Work out the finished part from the listing and answer in its coordinate system (mm). A direction names the side the tool comes from. Round coordinates to 2 decimals unless told otherwise and drop trailing zeros. Write each loop counter-clockwise with the first axis right and the second up, starting at its lowest first coordinate (ties: lowest second). Pieces come first, ordered by that corner, then holes. Notation, with made-up numbers: (43, 20) - (78, 20) arc R14 ccw to (78, 36) - close; hole circle Ø7 at (61.25, 37). An arc over 180 degrees is marked (long way). Answer as a JSON object with one key per item and string values.
```python
from build123d import *

# Parameters (mm, degrees)
SKETCH1_R           = 5.1
BOSS_EXTRUDE1_DEPTH = 10
SKETCH2_W           = 7.5
SKETCH2_H           = 16
BOSS_EXTRUDE2_DEPTH = 85
SKETCH3_W           = 29.2
SKETCH3_H           = 16
SKETCH3_R           = 5.1
BOSS_EXTRUDE3_DEPTH = 10
SKETCH4_W           = 29.2
SKETCH4_H           = 12
BOSS_EXTRUDE4_DEPTH = 10
CUT_EXTRUDE1_REACH  = 31.2
SKETCH6_W           = 29.2
SKETCH6_H           = 9.155809416
BOSS_EXTRUDE5_DEPTH = 28.3
SKETCH7_R           = 2.5
CUT_EXTRUDE2_DEPTH  = 20


with BuildPart() as part:
    # Sketch1 → Boss-Extrude1 (new body)
    with BuildSketch(Plane.XY):
        Polygon((-7.1, 8), (-14.6, 8), (-14.6, -8), (-7.1, -8), (7.1, -8), (14.6, -8), (14.6, 8), (7.1, 8), align=None)
        Circle(SKETCH1_R, mode=Mode.SUBTRACT)
    extrude(amount=BOSS_EXTRUDE1_DEPTH)

    # Sketch2 → Boss-Extrude2 (add)
    with BuildSketch(Plane.XY.offset(10)):
        with Locations((-10.85, 0)):
            Rectangle(SKETCH2_W, SKETCH2_H)
        with Locations((10.85, 0)):
            Rectangle(SKETCH2_W, SKETCH2_H)
    extrude(amount=BOSS_EXTRUDE2_DEPTH)

    # Sketch3 → Boss-Extrude3 (add)
    with BuildSketch(Plane.XY.offset(95)):
        Rectangle(SKETCH3_W, SKETCH3_H)
        Circle(SKETCH3_R, mode=Mode.SUBTRACT)
    extrude(amount=-BOSS_EXTRUDE3_DEPTH)

    # Sketch4 → Boss-Extrude4 (add)
    with BuildSketch(Plane.XY.offset(95)):
        with Locations((0, -14)):
            Rectangle(SKETCH4_W, SKETCH4_H)
    extrude(amount=-BOSS_EXTRUDE4_DEPTH)

    # Sketch5 → Cut-Extrude1 (cut, up to next)
    with BuildSketch(Plane(origin=(14.6, 0, 0), x_dir=(0, 0, -1), z_dir=(1, 0, 0)), mode=Mode.PRIVATE) as cut_extrude1_sk1:
        Polygon((-95, -12.5), (-89.748443463, -20), (-95, -20), align=None)
    cut_extrude1_tool1 = extrude(cut_extrude1_sk1.sketch, amount=-CUT_EXTRUDE1_REACH, mode=Mode.PRIVATE) & part.part
    add(cut_extrude1_tool1.solids().sort_by_distance((14.6, -17.5, 93.249481))[0], mode=Mode.SUBTRACT)

    # Sketch6 → Boss-Extrude5 (add)
    with BuildSketch(Plane(origin=(0, -48.747773592, 69.619035688), x_dir=(1, 0, 0), z_dir=(0, -0.573576436, 0.819152044))):
        with Locations((0, 39.672456192)):
            Rectangle(SKETCH6_W, SKETCH6_H)
    extrude(amount=BOSS_EXTRUDE5_DEPTH)

    # Sketch7 → Cut-Extrude2 (cut)
    with BuildSketch(Plane(origin=(0, -64.97998674, 92.801038541), x_dir=(1, 0, 0), z_dir=(0, -0.573576436, 0.819152044))):
        with Locations((-7.3, 39.672456192)):
            Circle(SKETCH7_R)
        with Locations((7.3, 39.672456192)):
            Circle(SKETCH7_R)
    extrude(amount=-CUT_EXTRUDE2_DEPTH, mode=Mode.SUBTRACT)


solid = part.part
```
Item 1: A cutting plane is placed at A-A (z = 68.5). Write down the section's boundary in (x, y), and give its area (3 significant figures).
Results found:
{"outline": "(-14.6, -8) - (-7.1, -8) - (-7.1, 8) - (-14.6, 8) - close; (7.1, -8) - (14.6, -8) - (14.6, 8) - (7.1, 8) - close", "area": "240 mm²"}
Item 2: Each of these flat-tipped pins is pushed along its axis until it touches: P1, Ø4, axis at x = -10, y = -21, coming from the +Z side; P2, Ø14.5, axis at x = -0.5, z = 39.5, coming from the -Y side; P3, Ø1.4, axis at x = -4, z = 88, coming from the -Y side; P4, Ø3, axis at x = -10, y = -6.5, coming from the -Z side. Where does it stop, or does it pass through?
Results found:
{"P1": "z = 110", "P2": "y = -8", "P3": "y = -20", "P4": "z = 0"}
Item 3: For faces 4 (the flat face through (7.1, 0, 47)), 5 (the flat face through (-10, 8, 47)), 6 (the flat face through (0, -9, 85)), 7 (the flat face through (-10, -8, 42)), 8 (the flat face through (-7.335, -20.982, 99.193)), determine the directions among +Z, -Z, +X, -X, +Y, -Y from which every point of the face is accessible in a straight line to the end or side of a thin tool.
Results found:
{"face 4": "+Y, -Y", "face 5": "+Z, -Z, +X, -X, +Y", "face 6": "-Y", "face 7": "-Z, +X, -X, -Y", "face 8": "none"}
Item 4: Determine the mould class of faces 1 (the flat face through (-0.204, -20.502, 106.429)), 2 (the cylindrical face through (2.4, -4.5, 90.1)), 3 (the flat face through (14.6, -2, 59)) for opening direction Y: pulls with the +Y half, pulls with the -Y half, needs draft (parallel to the pull), parting line crosses it, or undercut.
Results found:
{"face 1": "pulls with the +Y half", "face 2": "undercut", "face 3": "needs draft"}
Item 5: Consider line 1 along Z through (x, y) = (5.25, -3); line 2 along X through (y, z) = (3.5, 46); line 3 along Y through (x, z) = (0, 5.25). Determine where each line is inside the solid, lowest interval first.
Results found:
{"line 1": "0 to 10, 85 to 95", "line 2": "-14.6 to -7.1, 7.1 to 14.6", "line 3": "-8 to -5.1, 5.1 to 8"}
Item 6: A cutting plane is placed at D-D (z = 109). Give the number of separate pieces and of enclosed holes in the cut face, and give its area (3 significant figures).
Results found:
{"separate pieces": "1", "enclosed holes": "2", "area": "278 mm²"}
Item 7: A cutting plane is placed at C-C (y = 0). Write down the section's boundary in (x, z), and give its area (4 significant figures).
Results found:
{"outline": "(-14.6, 0) - (-5.1, 0) - (-5.1, 10) - (-7.1, 10) - (-7.1, 85) - (-5.1, 85) - (-5.1, 95) - (-14.6, 95) - close; (5.1, 0) - (14.6, 0) - (14.6, 95) - (5.1, 95) - (5.1, 85) - (7.1, 85) - (7.1, 10) - (5.1, 10) - close", "area": "1,505 mm²"}
Item 8: A cutting plane is placed at B-B (x = 0). Write down the section's boundary in (y, z), and give its area (3 significant figures).
Results found:
{"outline": "(-36.23, 112.93) - (-20, 89.75) - (-20, 85) - (-5.1, 85) - (-5.1, 95) - (-12.5, 95) - (-28.73, 118.18) - close; (-8, 0) - (-5.1, 0) - (-5.1, 10) - (-8, 10) - close; (5.1, 0) - (8, 0) - (8, 10) - (5.1, 10) - close; (5.1, 85) - (8, 85) - (8, 95) - (5.1, 95) - close", "area": "475 mm²"}
